```python
from build123d import *

# Parameters (mm, degrees)
F1_DEPTH = 10
F3_DEPTH = 674.322728
F6_DEPTH = 674.322728
F7_SIZE2 = 8
F7_SIZE  = 8


with BuildPart() as f1:
    # F0 (on Front) → F1 (new body)
    with BuildSketch(Plane.XZ):
        Polygon((-71, 100), (0, 0), (685, 0), (756, 100), align=None)
    extrude(amount=F1_DEPTH)

    # F2 (on face) → F3 (cut, through all)
    with BuildSketch(Plane(origin=(455.421847, 0, -323.349511), x_dir=(0, 1, 0), z_dir=(0.815383, 0, -0.578922))):
        Polygon((-10, 519.203269), (0, 519.203269), (0, 523.92737), (-15.178904, 523.92737), (-15.178904, 510.439725), (-10, 513.429767), align=None)
    extrude(amount=-F3_DEPTH, mode=Mode.SUBTRACT)

    # F5 (on face) → F6 (cut, through all)
    with BuildSketch(Plane(origin=(455.421847, 0, -323.349511), x_dir=(0, 1, 0), z_dir=(0.815383, 0, -0.578922))):
        Polygon((-196.915056, 209.646459), (-210.872175, 195.689339), (-196.915056, 195.689339), align=None)
    extrude(amount=-F6_DEPTH, mode=Mode.SUBTRACT)

    # F7
    f7_edges = [f1.edges().sort_by_distance(p)[0] for p in [
        (342.5, -10, 0),
    ]]
    chamfer(f7_edges, length=F7_SIZE, length2=F7_SIZE2)


solid = f1.part
```
Source: CAD feature listing. Evaluate the final solid. Frame: model axes, mm. Round coordinates to 2 decimals unless told otherwise and drop trailing zeros. Loops run counter-clockwise (first coordinate to the right, second up) from the corner with the lowest first, then second, coordinate; pieces in that order, holes last.
(1) Section query C-C (y = -4). Output: boundary loops of the cut face in (x, z), and give its area (3 significant figures).
From the geometry:
outline: (-71, 100) - (-1.42, 2) - (686.42, 2) - (756, 100) - close
area: 74,200 mm2
(2) Section query A-A (x = 558.5). Output: boundary loops of the cut face in (y, z).
From the geometry:
outline: (-10, 8) - (-2, 0) - (0, 0) - (0, 100) - (-10, 100) - close
(3) Material intervals for probe 1 along X at (y, z) = (-1, 8); probe 2 along X at (y, z) = (-9, 14.5) (3 decimals); probe 3 along Z at (x, y) = (56, -3.25), sorted ascending.
From the geometry:
probe 1: x = -5.68 to 690.68
probe 2: x = -10.295 to 695.295
probe 3: z = 1.25 to 100
(4) Contact query for flat-ended pins moving along their axis: pin 1 Ø3 at (x, y) = (596, -7) entering from -Z; pin 2 Ø1.5 at (y, z) = (-7, 72.5) entering from -X; pin 3 Ø5 at (y, z) = (-6, 82) entering from +X (3 decimals). Output: stop coordinate, or through.
From the geometry:
pin 1: stops at z = 3.5
pin 2: stops at x = -52.01
pin 3: stops at x = 744.995
(5) Section query B-B (z = 64). Output: boundary loops of the cut face in (x, y), and give its area (3 significant figures).
From the geometry:
outline: (-45.44, -10) - (730.44, -10) - (730.44, 0) - (-45.44, 0) - close
area: 7,760 mm2
